Autodesk Inventor part; units mm, degrees
ref_plane "Work Plane1" through (455, 0, 0) normal (-1, 0, 0) x (0, 0, 1)
ref_plane "Work Plane2" through (455, 0, 0) normal (-1, 0, 0) x (0, 0, 1)
ref_plane "Work Plane3" through (0, 0, 7.5) normal (0, 0, 1) x (1, 0, 0)
sketch "Sketch1" plane through (0, 0, 0) normal (0, 0, 1) x (1, 0, 0)
  line L0 (0, 0) -> (910, 0)
  line L1 (910, 0) -> (910, 55)
  line L2 (910, 55) -> (0, 55)
  line L3 (0, 55) -> (0, 0)
  dimension "d0" = 910
  dimension "d1" = 55
extrude "Extrusion1" add sketch "Sketch1" along normal blind 15
ref_plane "Work Plane1" through (455, 0, 0) normal (-1, 0, 0) x (0, 0, 1)
sketch "Sketch3" plane through (0, 0, 15) normal (0, 0, 1) x (1, 0, 0)
  line L0 (910, 55) -> (0, 55)
  line L1 (0, 55) -> (15, 55)
  line L2 (15, 55) -> (15, 27.5)
  line L3 (15, 27.5) -> (0, 27.5)
  line L4 (0, 27.5) -> (0, 55)
  line L5 (241.667, 55) -> (281.667, 55)
  line L6 (281.667, 55) -> (281.667, 27.5)
  line L7 (281.667, 27.5) -> (241.667, 27.5)
  line L8 (241.667, 27.5) -> (241.667, 55)
  line L9 (455, 55) -> (455, 32.488)
  line L10 (910, 55) -> (895, 55)
  line L11 (895, 55) -> (895, 27.5)
  line L12 (895, 27.5) -> (910, 27.5)
  line L13 (910, 27.5) -> (910, 55)
  line L14 (668.333, 55) -> (628.333, 55)
  line L15 (628.333, 55) -> (628.333, 27.5)
  line L16 (628.333, 27.5) -> (668.333, 27.5)
  line L17 (668.333, 27.5) -> (668.333, 55)
  point P0 (0, 0)
  point P1 (910, 0)
  point P2 (668.333, 55)
  point P3 (628.333, 55)
  dimension "d12" = 15
  dimension "d13" = 27.5
  dimension "d14" = 226.667
  dimension "d15" = 40
extrude "Extrusion2" cut sketch "Sketch3" against normal through all
ref_plane "Work Plane2" through (455, 0, 0) normal (-1, 0, 0) x (0, 0, 1)
ref_plane "Work Plane3" through (0, 0, 7.5) normal (0, 0, 1) x (1, 0, 0)
fillet "Fillet1" radius 3 6 edges at (895, 27.5, 7.5) (668.333, 27.5, 7.5) (628.333, 27.5, 7.5) (281.667, 27.5, 7.5) (241.667, 27.5, 7.5) (15, 27.5, 7.5)
properties part number "Length Board"
Model file for the job. Use its own axes, mm. A direction names the side the tool comes from. Give positions to 0.01 mm unless a question says otherwise; leave off trailing zeros. Write each loop counter-clockwise with the first axis right and the second up, starting at its lowest first coordinate (ties: lowest second). Pieces come first, ordered by that corner, then holes. Notation, with made-up numbers: (-15, 16) -> (-8, 16) arc R12 ccw to (-8, 22) -> close; hole circle Ø7 at (61, 83.5). An arc over 180 degrees is marked (long way). Write item = value, one per line.
(1) Slice it at A-A, the plane y = 42.5. Give the cut face in (x, z).
Determined:
outline = (15, 0) -> (241.67, 0) -> (241.67, 15) -> (15, 15) -> close; (281.67, 0) -> (628.33, 0) -> (628.33, 15) -> (281.67, 15) -> close; (668.33, 0) -> (895, 0) -> (895, 15) -> (668.33, 15) -> close
(2) Mould opens along X. For faces 4 (the face through (449, 28, 0)), 5 (the face through (895, 43, 8)), 6 (the face through (281.667, 43, 8)) say: released by +X, released by -X, zero draft, split by the parting line, or undercut.
Determined:
face_4 = zero draft
face_5 = released by +X
face_6 = undercut
(3) Flat gauge pins, fed straight in: P1, Ø4.5, axis at y = 46.5, z = 10, coming from the +X side; P2, Ø3, axis at y = 41, z = 3.5, coming from the -X side; P3, Ø7.5, axis at x = 647.5, z = 9, coming from the +Y side. Where does each tip first touch, or does it go through?
Determined:
P1 = 895
P2 = 15
P3 = 27.5
(4) Slice it at B-B, the plane z = 10.25. Give the cut face in (x, y), then the cut area to 3 significant figures.
Determined:
outline = (0, 0) -> (910, 0) -> (910, 27.5) -> (898, 27.5) arc R3 cw to (895, 30.5) -> (895, 55) -> (668.33, 55) -> (668.33, 30.5) arc R3 cw to (665.33, 27.5) -> (631.33, 27.5) arc R3 cw to (628.33, 30.5) -> (628.33, 55) -> (281.67, 55) -> (281.67, 30.5) arc R3 cw to (278.67, 27.5) -> (244.67, 27.5) arc R3 cw to (241.67, 30.5) -> (241.67, 55) -> (15, 55) -> (15, 30.5) arc R3 cw to (12, 27.5) -> (0, 27.5) -> close
area = 47,000 mm2
(5) Probe line 1 along X through (y, z) = (50, 4.75); line 2 along Y through (x, z) = (243, 11.75). List the from-to ranges inside material, lowest first.
Determined:
line_1 = 15 to 241.67, 281.67 to 628.33, 668.33 to 895
line_2 = 0 to 28.01
(6) Tool access for faces 1 (the face through (15, 43, 8)), 2 (the face through (668.333, 43, 8)), 3 (the face through (783, 55, 7)): list every direction of +Z, -Z, +X, -X, +Y, -Y with a clear straight run to the whole face (end or side of a thin tool).
Determined:
face_1 = +Z, -Z, -X, +Y
face_2 = +Z, -Z, +Y
face_3 = +Z, -Z, +X, -X, +Y
